Work out the finished part from the listing and answer in its coordinate system (mm). A direction names the side the tool comes from. Coordinates: 2 decimals unless noted, no trailing zeros. Write each loop counter-clockwise with the first axis right and the second up, starting at its lowest first coordinate (ties: lowest second). Pieces come first, ordered by that corner, then holes. Notation, with made-up numbers: (78.5, 49) - (134.5, 49) arc R19 ccw to (134.5, 78) - close; hole circle Ø10 at (-15, 5). An arc over 180 degrees is marked (long way). Use one line per item in the form item = value. Start each with the question number.
Item 1: A cutting plane is placed at B-B (x = 37). Write down the section's boundary in (y, z), then the cut area to 3 significant figures.
Item 2: Given pin 1 (3.5 mm diameter, centred on x = 34, z = 6.5, fed in from -Y); pin 2 (0.9 mm diameter, centred on x = 17.5, y = 24, fed in from -Z); pin 3 (10 mm diameter, centred on x = 6.5, y = 21.5, fed in from -Z); pin 4 (2.5 mm diameter, centred on x = 37, y = 23.82, fed in from +Z), each flat-ended and moving along its own axis, determine where each tip first touches the part or whether it passes through.
Item 3: Consider probe 1 along Y at (x, z) = (17, 2.2); probe 2 along X at (y, z) = (1.75, 5); probe 3 along X at (y, z) = (24.25, 30.25). Determine where each line is inside the solid, lowest interval first.
Item 4: A cutting plane is placed at C-C (z = 11). Write down the section's boundary in (x, y).
Item 5: A cutting plane is placed at A-A (y = 12). Write down the section's boundary in (x, z), then the cut area to 3 significant figures.
Item 6: For faces 5 (the cylindrical face through (38.45, 23.88, 2.46)), 6 (the flat face through (17, 24, 42)), 7 (the flat face through (27, 21, 6)), determine the directions among +Z, -Z, +X, -X, +Y, -Y from which every point of the face is accessible in a straight line to the end or side of a thin tool.
Item 7: Determine the mould class of faces 1 (the cylindrical face through (19.77, 22.85, 26.79)), 2 (the flat face through (2, 0, 6)), 3 (the flat face through (54, 14, 6)), 4 (the cylindrical face through (15.617, 24.252, 2.465)) for opening direction X: released by +X, released by -X, zero draft, split by the parting line, or undercut.
from build123d import *

# Parameters (mm, degrees)
BOSS_EXTRUDE1_DEPTH = 12
SKETCH2_R           = 3
BOSS_EXTRUDE2_DEPTH = 30
CUT_EXTRUDE1_REACH  = 29
SKETCH3_R           = 0.75
SKETCH4_R           = 1.45
CUT_EXTRUDE2_DEPTH  = 5


with BuildPart() as part:
    # Sketch1 → Boss-Extrude1 (new body)
    with BuildSketch(Plane.XY):
        Polygon((0, 0), (0, 27), (54, 27), (54, 0), (51, 0), (51, 21), (3, 21), (3, 0), align=None)
    extrude(amount=BOSS_EXTRUDE1_DEPTH)

    # Sketch2 → Boss-Extrude2 (add)
    with BuildSketch(Plane.XY.offset(12)):
        with Locations((17, 24)):
            Circle(SKETCH2_R)
    extrude(amount=BOSS_EXTRUDE2_DEPTH)

    # Sketch3 → Cut-Extrude1 (cut, up to next)
    with BuildSketch(Plane(origin=(0, 27, 0), x_dir=(1, 0, 0), z_dir=(0, 1, 0)), mode=Mode.PRIVATE) as cut_extrude1_sk1:
        with Locations((16.346450023, -38.25)):
            Circle(SKETCH3_R)
    cut_extrude1_tool1 = extrude(cut_extrude1_sk1.sketch, amount=-CUT_EXTRUDE1_REACH, mode=Mode.PRIVATE) & part.part
    add(cut_extrude1_tool1.solids().sort_by_distance((16.34645, 27, 38.25))[0], mode=Mode.SUBTRACT)
    # Sketch3 → Cut-Extrude1 (cut, up to next)
    with BuildSketch(Plane(origin=(0, 27, 0), x_dir=(1, 0, 0), z_dir=(0, 1, 0)), mode=Mode.PRIVATE) as cut_extrude1_sk2:
        with Locations((16.346450023, -34.25)):
            Circle(SKETCH3_R)
    cut_extrude1_tool2 = extrude(cut_extrude1_sk2.sketch, amount=-CUT_EXTRUDE1_REACH, mode=Mode.PRIVATE) & part.part
    add(cut_extrude1_tool2.solids().sort_by_distance((16.34645, 27, 34.25))[0], mode=Mode.SUBTRACT)
    # Sketch3 → Cut-Extrude1 (cut, up to next)
    with BuildSketch(Plane(origin=(0, 27, 0), x_dir=(1, 0, 0), z_dir=(0, 1, 0)), mode=Mode.PRIVATE) as cut_extrude1_sk3:
        with Locations((16.346450023, -30.25)):
            Circle(SKETCH3_R)
    cut_extrude1_tool3 = extrude(cut_extrude1_sk3.sketch, amount=-CUT_EXTRUDE1_REACH, mode=Mode.PRIVATE) & part.part
    add(cut_extrude1_tool3.solids().sort_by_distance((16.34645, 27, 30.25))[0], mode=Mode.SUBTRACT)
    # Sketch3 → Cut-Extrude1 (cut, up to next)
    with BuildSketch(Plane(origin=(0, 27, 0), x_dir=(1, 0, 0), z_dir=(0, 1, 0)), mode=Mode.PRIVATE) as cut_extrude1_sk4:
        with Locations((16.346450023, -26.25)):
            Circle(SKETCH3_R)
    cut_extrude1_tool4 = extrude(cut_extrude1_sk4.sketch, amount=-CUT_EXTRUDE1_REACH, mode=Mode.PRIVATE) & part.part
    add(cut_extrude1_tool4.solids().sort_by_distance((16.34645, 27, 26.25))[0], mode=Mode.SUBTRACT)

    # Sketch4 → Cut-Extrude2 (cut)
    with BuildSketch(Plane(origin=(0, 0, 0), x_dir=(-1, 0, 0), z_dir=(0, 0, -1))):
        with Locations((-37, 23.816903441)):
            Circle(SKETCH4_R)
        with Locations((-17, 23.816903441)):
            Circle(SKETCH4_R)
    extrude(amount=-CUT_EXTRUDE2_DEPTH, mode=Mode.SUBTRACT)


solid = part.part
Answer:
q1.outline = (21, 0) - (22.37, 0) - (22.37, 5) - (25.27, 5) - (25.27, 0) - (27, 0) - (27, 12) - (21, 12) - close
q1.area = 57.5 mm²
q2.pin_1 = 21
q2.pin_2 = 5
q2.pin_3 = 0
q2.pin_4 = 12
q3.probe_1 = 21 to 22.37, 25.27 to 27
q3.probe_2 = 0 to 3, 51 to 54
q3.probe_3 = 14.01 to 15.6, 17.1 to 19.99
q4.outline = (0, 0) - (3, 0) - (3, 21) - (51, 21) - (51, 0) - (54, 0) - (54, 27) - (0, 27) - close
q5.outline = (0, 0) - (3, 0) - (3, 12) - (0, 12) - close; (51, 0) - (54, 0) - (54, 12) - (51, 12) - close
q5.area = 72.0 mm²
q6.face_5 = -Z
q6.face_6 = +Z, +X, -X, +Y, -Y
q6.face_7 = +Z, -Z, -Y
q7.face_1 = split by the parting line
q7.face_2 = zero draft
q7.face_3 = released by +X
q7.face_4 = undercut
